Part model, mm, in its own coordinate system. Round coordinates to 2 decimals unless told otherwise and drop trailing zeros. Write each loop counter-clockwise with the first axis right and the second up, starting at its lowest first coordinate (ties: lowest second). Pieces come first, ordered by that corner, then holes.
```python
from build123d import *

# Parameters (mm, degrees)
SKETCH_1_W             = 28
SKETCH_1_H             = 3
EXTRUDE_1_DEPTH        = 337
SKETCH_2_R             = 7.5
SKETCH_2_R_2           = 1.5
CUT_EXTRUDE_1_DEPTH    = 400
SKETCH_3_R             = 1.5
SKETCH_3_W             = 18
SKETCH_3_H             = 22
CUT_EXTRUDE_2_DEPTH    = 10
SKETCH_4_R             = 1.5
CUT_EXTRUDE_3_DEPTH    = 10
SKETCH_5_R             = 1.5
CUT_EXTRUDE_4_DEPTH    = 10
FILLET_1_R             = 2
FILLET_3_R             = 3
PATTERN_LINEAR_1_COUNT = 2
PATTERN_LINEAR_1_PITCH = 211.46


with BuildPart() as part:
    # 草图1 → 凸台-拉伸1 (new body)
    with BuildSketch(Plane.XY):
        Rectangle(SKETCH_1_W, SKETCH_1_H)
    extrude(amount=EXTRUDE_1_DEPTH)

    # 草图2 → 切除-拉伸1 (cut)
    with BuildSketch(Plane.XZ.offset(1.5)):
        with Locations((0, 164.5)):
            Circle(SKETCH_2_R)
        with Locations((-9.5, 179)):
            Circle(SKETCH_2_R_2)
        with Locations((9.5, 179)):
            Circle(SKETCH_2_R_2)
        with Locations((9.5, 150)):
            Circle(SKETCH_2_R_2)
        with Locations((-9.5, 150)):
            Circle(SKETCH_2_R_2)
    extrude(amount=-CUT_EXTRUDE_1_DEPTH, mode=Mode.SUBTRACT)

    # 草图3 → 切除-拉伸2 (cut)
    with BuildSketch(Plane(origin=(0, 1.5, 0), x_dir=(1, 0, 0), z_dir=(0, 1, 0))):
        with Locations(Location((11.5, -3.5, 0), (0, 0, 180))):
            Circle(SKETCH_3_R)
        with Locations(Location((-11.5, -3.5, 0), (0, 0, 180))):
            Circle(SKETCH_3_R)
        with Locations(Location((-11.5, -36.5, 0), (0, 0, 180))):
            Circle(SKETCH_3_R)
        with Locations(Location((11.5, -36.5, 0), (0, 0, 180))):
            Circle(SKETCH_3_R)
        with Locations((0, -20)):
            Rectangle(SKETCH_3_W, SKETCH_3_H)
    extrude(amount=-CUT_EXTRUDE_2_DEPTH, mode=Mode.SUBTRACT)

    # 草图4 → 切除-拉伸3 (cut)
    with BuildSketch(Plane(origin=(0, 1.5, 0), x_dir=(1, 0, 0), z_dir=(0, 1, 0))):
        with Locations(Location((7, -332, 0), (0, 0, 180))):
            Circle(SKETCH_4_R)
        with Locations(Location((-7, -332, 0), (0, 0, 180))):
            Circle(SKETCH_4_R)
    extrude(amount=-CUT_EXTRUDE_3_DEPTH, mode=Mode.SUBTRACT)

    # 草图5 → 切除-拉伸4 (cut)
    with BuildSketch(Plane.XZ.offset(1.5)):
        with Locations((-10.5, 264.73)):
            Circle(SKETCH_5_R)
        with Locations((-10.5, 275.73)):
            Circle(SKETCH_5_R)
        with Locations((10.5, 275.73)):
            Circle(SKETCH_5_R)
        with Locations((10.5, 264.73)):
            Circle(SKETCH_5_R)
    cut_extrude_4 = extrude(amount=-CUT_EXTRUDE_4_DEPTH, mode=Mode.SUBTRACT)

    # 圆角1
    fillet_1_edges = [part.edges().sort_by_distance(p)[0] for p in [
        (-14, 0, 337),
        (14, 0, 337),
        (-14, 0, 0),
        (14, 0, 0),
    ]]
    fillet(fillet_1_edges, radius=FILLET_1_R)

    # 圆角3
    fillet_3_edges = [part.edges().sort_by_distance(p)[0] for p in [
        (9, 0, 9),
        (9, 0, 31),
        (-9, 0, 31),
        (-9, 0, 9),
    ]]
    fillet(fillet_3_edges, radius=FILLET_3_R)

    # 阵列(线性)1: 切除-拉伸4 ×2
    with Locations(*[(0, 0, -i * PATTERN_LINEAR_1_PITCH) for i in range(1, PATTERN_LINEAR_1_COUNT)]):
        add(cut_extrude_4, mode=Mode.SUBTRACT)


solid = part.part
```
Q1. Cut at B-B on y = -0.35. State how many separate pieces and enclosed holes the cut face has, plus the area to 3 significant figures.
Values follow:
separate pieces: 1
enclosed holes: 20
area: 8,740 mm2
Q2. Drop a flat-ended pin along its axis: pin 1 (5 mm diameter, centred on x = -10.5, z = 53.27, fed in from -Y). Give the stop position or say it passes through.
Values follow:
pin 1: stops at y = -1.5
Q3. Mould opens along X. For faces 1 (the flat face through (-10, -1.5, 166)), 2 (the cylindrical face through (-0.976, -0.021, 171.936)) say: +X half, -X half, draft (parallel to the pull), parting line (faces both ways), or undercut.
Values follow:
face 1: draft
face 2: undercut
Q4. Wall check: L1, parallel to Z at x = 0.75, y = -0.2; L2, parallel to X at y = -0.4, z = 275.73; L3, parallel to X at y = -0.1, z = 179. Give the ranges that are in metal, low to high.
Values follow:
L1: z = 0 to 9, 31 to 157.04, 171.96 to 337
L2: x = -14 to -12, -9 to 9, 12 to 14
L3: x = -14 to -11, -8 to 8, 11 to 14
Q5. Cut at A-A on x = 0. Write the cut outline in (y, z), plus the area to 3 significant figures.
Values follow:
outline: (-1.5, 0) - (1.5, 0) - (1.5, 9) - (-1.5, 9) - close; (-1.5, 31) - (1.5, 31) - (1.5, 157) - (-1.5, 157) - close; (-1.5, 172) - (1.5, 172) - (1.5, 337) - (-1.5, 337) - close
area: 900 mm2
